Can you work these out from the model? Positions are in its coordinate system, mm. Face numbers are marked on the shaded views. A direction names the side the tool comes from. Give positions to 0.01 mm unless a question says otherwise; leave off trailing zeros. Order: outer loops, then holes, each group sorted by start corner. A loop starts at its lowest first (then second) coordinate and runs counter-clockwise, first axis right, second up.
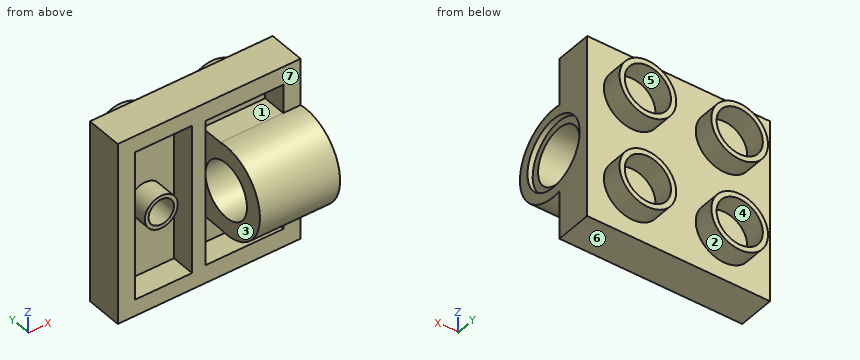
```python
from build123d import *

# Parameters (mm, degrees)
SKETCH1_W               = 15.8
SKETCH1_H               = 15.8
BOSS_EXTRUDE1_DEPTH     = 7.71
SKETCH2_R               = 2.99
CUT_EXTRUDE1_DEPTH      = 0.45
SKETCH3_R               = 2.375
CUT_EXTRUDE2_DEPTH      = 6.56
CUT_EXTRUDE4_DEPTH      = 20.274182214
CUT_EXTRUDE4_DEPTH_BACK = 20.274182214
CUT_EXTRUDE5_DEPTH      = 20.274182214
CUT_EXTRUDE5_DEPTH_BACK = 8.87
CUT_EXTRUDE6_DEPTH      = 2.07
SKETCH10_W              = 5.44
SKETCH10_H              = 0.215050188
CUT_EXTRUDE8_DEPTH      = 2.07
SKETCH11_W              = 5.44
SKETCH11_H              = 0.461737218
CUT_EXTRUDE9_DEPTH      = 2.07
SKETCH12_W              = 4.93
SKETCH12_H              = 12.94
CUT_EXTRUDE10_DEPTH     = 2.07
SKETCH13_R              = 1.425
SKETCH13_R_2            = 1.1
BOSS_EXTRUDE2_DEPTH     = 1.87
SKETCH14_R              = 2.45
SKETCH14_R_2            = 2
BOSS_EXTRUDE3_DEPTH     = 1.79


with BuildPart() as part:
    # Sketch1 → Boss-Extrude1 (new body)
    with BuildSketch(Plane(origin=(0, 0, 0), x_dir=(1, 0, 0), z_dir=(0, 1, 0))):
        Rectangle(SKETCH1_W, SKETCH1_H)
    extrude(amount=-BOSS_EXTRUDE1_DEPTH)

    # Sketch2 → Cut-Extrude1 (cut)
    with BuildSketch(Plane(origin=(7.9, 0, 0), x_dir=(0, 0, -1), z_dir=(1, 0, 0))):
        with Locations((-0.04, -3.855)):
            Circle(SKETCH2_R)
    extrude(amount=-CUT_EXTRUDE1_DEPTH, mode=Mode.SUBTRACT)

    # Sketch3 → Cut-Extrude2 (cut)
    with BuildSketch(Plane(origin=(7.45, 0, 0), x_dir=(0, 0, -1), z_dir=(1, 0, 0))):
        with Locations((-0.04, -3.855)):
            Circle(SKETCH3_R)
    extrude(amount=-CUT_EXTRUDE2_DEPTH, mode=Mode.SUBTRACT)

    # Sketch4 → Cut-Extrude4 (cut, two sides: drawn at the far end of the back side and taken through both)
    with BuildSketch(Plane(origin=(7.9, 0, 0), x_dir=(0, 0, -1), z_dir=(1, 0, 0)).offset(-CUT_EXTRUDE4_DEPTH_BACK)):
        with BuildLine():
            Line((-50.773144054, -3.18), (-7.9, -3.18))
            Line((-7.9, -3.18), (-3.835444638, -3.18))
            ThreePointArc((-3.835444638, -3.18), (-0.04, -7.71), (3.755444638, -3.18))
            Line((3.755444638, -3.18), (7.9, -3.18))
            Line((7.9, -3.18), (50.773144054, -3.18))
            Line((50.773144054, -3.18), (50.773144054, -88.926288108))
            Line((50.773144054, -88.926288108), (-50.773144054, -88.926288108))
            Line((-50.773144054, -88.926288108), (-50.773144054, -3.18))
        make_face()
    extrude(amount=CUT_EXTRUDE4_DEPTH + CUT_EXTRUDE4_DEPTH_BACK, mode=Mode.SUBTRACT)

    # Sketch6 → Cut-Extrude5 (cut, two sides: drawn at the far end of the back side and taken through both)
    with BuildSketch(Plane.ZY.offset(7.9).offset(-CUT_EXTRUDE5_DEPTH_BACK)):
        Polygon((-38.914265028, -3.18), (-3.755444638, -3.18), (3.835444638, -3.18), (38.994265028, -3.18), (38.994265028, -73.49764078), (-38.914265028, -73.49764078), align=None)
    extrude(amount=CUT_EXTRUDE5_DEPTH + CUT_EXTRUDE5_DEPTH_BACK, mode=Mode.SUBTRACT)

    # Sketch7 → Cut-Extrude6 (cut)
    with BuildSketch(Plane.XZ.offset(3.18)):
        Polygon((6.41, 6.33), (-0.33, 6.33), (-0.33, -6.33), (6.41, -6.33), (6.41, -4.217181856), (0.97, -4.217181856), (0.97, 4.050494826), (6.41, 4.050494826), align=None)
    extrude(amount=-CUT_EXTRUDE6_DEPTH, mode=Mode.SUBTRACT)

    # Sketch10 → Cut-Extrude8 (cut)
    with BuildSketch(Plane.XZ.offset(3.18)):
        with Locations((3.69, 3.942969732)):
            Rectangle(SKETCH10_W, SKETCH10_H)
    extrude(amount=-CUT_EXTRUDE8_DEPTH, mode=Mode.SUBTRACT)

    # Sketch11 → Cut-Extrude9 (cut)
    with BuildSketch(Plane.XZ.offset(3.18)):
        with Locations((3.69, -3.986313247)):
            Rectangle(SKETCH11_W, SKETCH11_H)
    extrude(amount=-CUT_EXTRUDE9_DEPTH, mode=Mode.SUBTRACT)

    # Sketch12 → Cut-Extrude10 (cut)
    with BuildSketch(Plane.XZ.offset(3.18)):
        with Locations((-3.945, 0)):
            Rectangle(SKETCH12_W, SKETCH12_H)
    extrude(amount=-CUT_EXTRUDE10_DEPTH, mode=Mode.SUBTRACT)

    # Sketch13 → Boss-Extrude2 (add)
    with BuildSketch(Plane.XZ.offset(1.11)):
        with Locations(Location((-3.985, -0.04, 0), (0, 0, 90))):
            Circle(SKETCH13_R)
        with Locations(Location((-3.985, -0.04, 0), (0, 0, 90))):
            Circle(SKETCH13_R_2, mode=Mode.SUBTRACT)
    extrude(amount=BOSS_EXTRUDE2_DEPTH)

    # Sketch14 → Boss-Extrude3 (add)
    # profile 1 of 4: a face of its own
    with BuildSketch(Plane(origin=(0, 0, 0), x_dir=(1, 0, 0), z_dir=(0, 1, 0))):
        with Locations(Location((-3.93, 3.93, 0), (0, 0, 90))):
            Circle(SKETCH14_R)
        with Locations(Location((-3.93, 3.93, 0), (0, 0, 90))):
            Circle(SKETCH14_R_2, mode=Mode.SUBTRACT)
    # profile 2 of 4: a face of its own
    with BuildSketch(Plane(origin=(0, 0, 0), x_dir=(1, 0, 0), z_dir=(0, 1, 0))):
        with Locations(Location((4.01, 3.93, 0), (0, 0, 90))):
            Circle(SKETCH14_R)
        with Locations(Location((4.01, 3.93, 0), (0, 0, 90))):
            Circle(SKETCH14_R_2, mode=Mode.SUBTRACT)
    # profile 3 of 4: a face of its own
    with BuildSketch(Plane(origin=(0, 0, 0), x_dir=(1, 0, 0), z_dir=(0, 1, 0))):
        with Locations(Location((-3.93, -4.01, 0), (0, 0, 90))):
            Circle(SKETCH14_R)
        with Locations(Location((-3.93, -4.01, 0), (0, 0, 90))):
            Circle(SKETCH14_R_2, mode=Mode.SUBTRACT)
    # profile 4 of 4: a face of its own
    with BuildSketch(Plane(origin=(0, 0, 0), x_dir=(1, 0, 0), z_dir=(0, 1, 0))):
        with Locations(Location((4.01, -4.01, 0), (0, 0, 90))):
            Circle(SKETCH14_R)
        with Locations(Location((4.01, -4.01, 0), (0, 0, 90))):
            Circle(SKETCH14_R_2, mode=Mode.SUBTRACT)
    extrude(amount=BOSS_EXTRUDE3_DEPTH)


solid = part.part
```
1) Suppose I cut it at C-C (y = -2.25). Please give me the cut outline in (x, z) (3 decimals).
2) We'd pull the mould along Z, two halves only. Please class the marked faces 4, 5, 6 and 7: +Z half, -Z half, draft (parallel to the pull), parting line (faces both ways), or undercut.
3) Suppose I cut it at A-A (y = 0.5). Please give me the cut outline in (x, z).
4) Suppose I cut it at B-B (z = -0.04). Please give me the cut outline in (x, y) (3 decimals).
5) Which directions (+Z, -Z, +X, -X, +Y, -Y) give clear straight access to the entire face, cutting with the end or side of a thin tool? Please do the marked faces 1, 2 and 3.
6) If I drill on line 1 (X direction, y = 0.9, z = -3.93); line 2 (Z direction, x = 4.25, y = 0.25); line 3 (Z direction, x = -2.75, y = 1), over which ranges is the centre line in solid material (lowest first)?
7) I'm going to push flat-ended pins straight in: pin 1 Ø5 at (x, z) = (2, 5.5) entering from -Y; pin 2 Ø2.5 at (y, z) = (-2.5, 1) entering from +X; pin 3 Ø1.7 at (y, z) = (-2.5, 0.5) entering from +X; pin 4 Ø1.8 at (y, z) = (-4.5, -1) entering from +X. Where does each tip first touch, or does it pass through?
Results:
1. outline: (-7.9, -7.9) - (7.9, -7.9) - (7.9, -2.483) - (7.45, -2.483) - (7.45, -1.711) - (0.97, -1.711) - (0.97, -3.755) - (6.41, -3.755) - (6.41, -6.33) - (-0.33, -6.33) - (-0.33, 6.33) - (6.41, 6.33) - (6.41, 3.835) - (0.97, 3.835) - (0.97, 1.791) - (7.45, 1.791) - (7.45, 2.563) - (7.9, 2.563) - (7.9, 7.9) - (-7.9, 7.9) - close; circle Ø2.85 at (-3.985, -0.04); hole (-6.41, -6.47) - (-1.48, -6.47) - (-1.48, 6.47) - (-6.41, 6.47) - close; hole circle Ø2.2 at (-3.985, -0.04)
2. face 4: undercut
2. face 5: undercut
2. face 6: -Z half
2. face 7: draft
3. outline: circle Ø4.9 at (-3.93, -3.93); circle Ø4.9 at (-3.93, 4.01); circle Ø4.9 at (4.01, -3.93); circle Ø4.9 at (4.01, 4.01); hole circle Ø4 at (-3.93, -3.93); hole circle Ø4 at (-3.93, 4.01); hole circle Ø4 at (4.01, -3.93); hole circle Ø4 at (4.01, 4.01)
4. outline: (-7.9, -3.18) - (-6.41, -3.18) - (-6.41, -1.11) - (-5.41, -1.11) - (-5.41, -2.98) - (-5.085, -2.98) - (-5.085, -1.11) - (-2.885, -1.11) - (-2.885, -2.98) - (-2.56, -2.98) - (-2.56, -1.11) - (-1.48, -1.11) - (-1.48, -3.18) - (-0.33, -3.18) - (-0.33, -1.11) - (0.97, -1.11) - (0.97, -1.481) - (7.45, -1.481) - (7.45, -0.866) - (7.9, -0.866) - (7.9, 0) - (-7.9, 0) - close; (0.97, -7.709) - (7.9, -7.709) - (7.9, -6.844) - (7.45, -6.844) - (7.45, -6.229) - (0.97, -6.229) - close
5. face 1: none
5. face 2: +Y
5. face 3: -Y
6. line 1: x = -6.38 to -5.93, -1.93 to -1.48, 1.56 to 2.01, 6.01 to 6.46
6. line 2: z = -6.37 to -5.92, -1.94 to -1.49, 1.57 to 2.02, 6 to 6.45
6. line 3: z = -6.08 to -5.54, -2.32 to -1.78, 1.86 to 2.4, 5.62 to 6.16
7. pin 1: stops at y = -6.32
7. pin 2: stops at x = 7.45
7. pin 3: stops at x = -0.33
7. pin 4: passes through
